Input: dimensioned drawing with shaded views. Units: mm. Origin: part minimum x, y, z. Coordinates: 2 decimals unless noted, no trailing zeros. Order: outer loops, then holes, each group sorted by start corner. A loop starts at its lowest first (then second) coordinate and runs counter-clockwise, first axis right, second up. Notation, with made-up numbers: (40.25, 4.25) - (58.25, 4.25) arc R25 ccw to (58.25, 17.25) - close; hole circle Ø5 at (57, -10.5). An arc over 180 degrees is marked (long way). One line per question, with ' | ' between items. Start each with the question number.
(1) Section B-B (x = 27.5). Return the cut outline in (y, z), then the cut area to 3 significant figures.
(2) Section C-C (z = 36). Return the cut outline in (x, y).
(3) Contact query for flat-ended pins moving along their axis: P1, Ø4, axis at y = 3, z = 62.5, coming from the -X side; P2, Ø8, axis at x = 18, z = 169, coming from the +Y side; P3, Ø1, axis at y = 4, z = 151, coming from the +X side (3 decimals). Output: stop coordinate, or through.
(4) Line query: line 1 along Z through (x, y) = (8.25, 5.5); line 2 along X through (y, z) = (5.5, 160.5) (1 decimal); line 3 along Y through (x, z) = (15.5, 117.5) (1 decimal). Output: solid intervals per line, ascending.
(5) Section A-A (y = 5). Return the cut outline in (x, z).
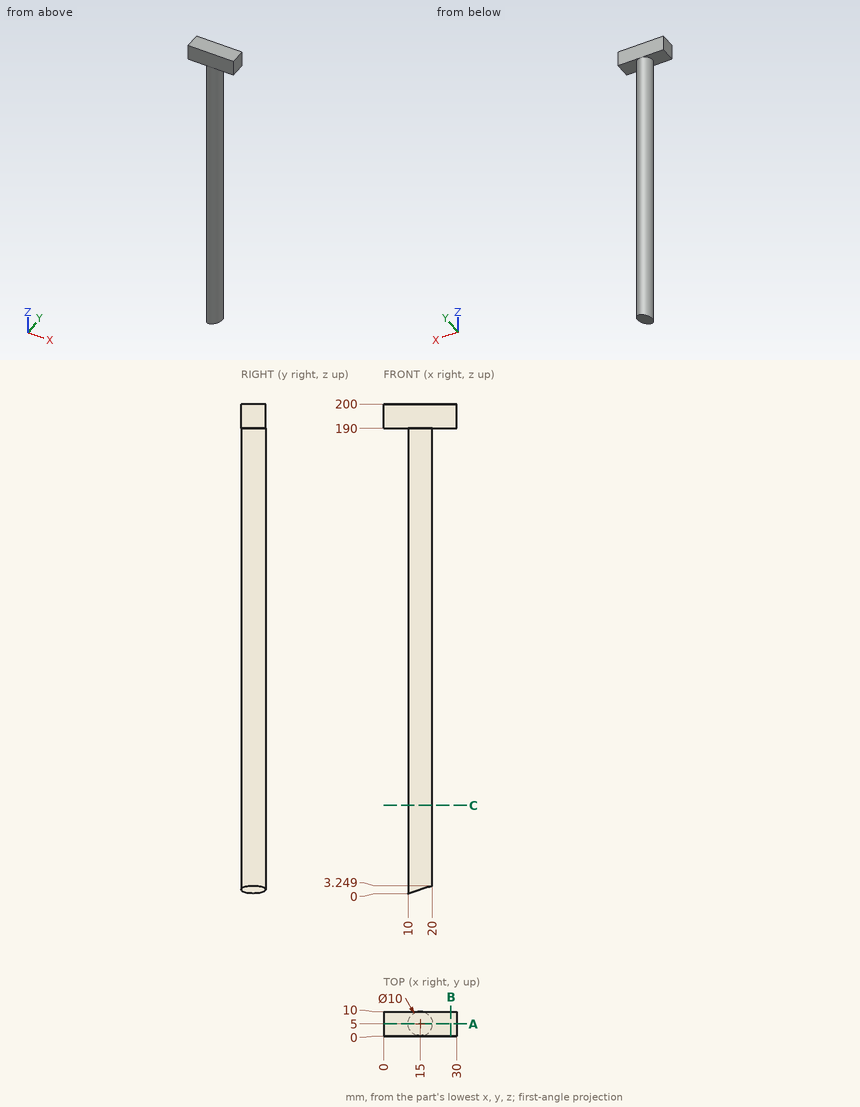
Response values:
1) outline: (0, 190) - (10, 190) - (10, 200) - (0, 200) - close | area: 100 mm²
2) outline: circle Ø10 at (15, 5)
3) P1: stops at x = 10 | P2: stops at y = 10 | P3: stops at x = 19.975
4) line 1: z = 190 to 200 | line 2: x = 10 to 20 | line 3: y = 0 to 10
5) outline: (0, 190) - (10, 190) - (10, 0) - (20, 3.25) - (20, 190) - (30, 190) - (30, 200) - (0, 200) - close
